```python
from build123d import *
from OCP.BRepFilletAPI import BRepFilletAPI_MakeChamfer

# Parameters (mm, degrees)
SCHIZZO1_W                   = 34
SCHIZZO1_H                   = 30
ESTRUSIONE_ESTRUSIONE1_DEPTH = 22
SCHIZZO2_W                   = 1
SCHIZZO2_H                   = 14.267949192
TAGLIO_ESTRUSIONE1_DEPTH     = 37.193922142
SCHIZZO3_W                   = 10.8571
SCHIZZO3_H                   = 4
TAGLIO_ESTRUSIONE2_DEPTH     = 37.193922142
SCHIZZO4_W                   = 11.8571
SCHIZZO4_H                   = 4
TAGLIO_ESTRUSIONE3_DEPTH     = 37.193922142
SCHIZZO5_W                   = 1
SCHIZZO5_H                   = 10.267949192
TAGLIO_ESTRUSIONE4_DEPTH     = 37.193922142
SCHIZZO6_W                   = 15.2
SCHIZZO6_H                   = 0.4
TAGLIO_ESTRUSIONE5_DEPTH     = 37.193922142
SFORMO1_ANGLE                = 60
SFORMO2_ANGLE                = 60
SFORMO3_ANGLE                = 45
SFORMO4_ANGLE                = 45
SMUSSO1_SIZE                 = 0.230940108
SMUSSO1_SIZE2                = 0.4
SMUSSO2_SIZE                 = 0.379
SMUSSO3_SIZE                 = 1


with BuildPart() as part:
    # Schizzo1 → Estrusione-Estrusione1 (new body)
    with BuildSketch(Plane(origin=(0, 11, 0), x_dir=(1, 0, 0), z_dir=(0, 1, 0))):
        with Locations((0, -15)):
            Rectangle(SCHIZZO1_W, SCHIZZO1_H)
    extrude(amount=-ESTRUSIONE_ESTRUSIONE1_DEPTH)

    # Schizzo2 → Taglio-Estrusione1 (cut, through all)
    with BuildSketch(Plane.XY.offset(30)):
        with Locations((16.5, -3.866025404)):
            Rectangle(SCHIZZO2_W, SCHIZZO2_H)
    extrude(amount=-TAGLIO_ESTRUSIONE1_DEPTH, mode=Mode.SUBTRACT)

    # Schizzo3 → Taglio-Estrusione2 (cut, through all)
    with BuildSketch(Plane.XY.offset(30)):
        with Locations((10.57145, -9)):
            Rectangle(SCHIZZO3_W, SCHIZZO3_H)
    extrude(amount=-TAGLIO_ESTRUSIONE2_DEPTH, mode=Mode.SUBTRACT)

    # Schizzo4 → Taglio-Estrusione3 (cut, through all)
    with BuildSketch(Plane.XY.offset(30)):
        with Locations((-11.07145, -9)):
            Rectangle(SCHIZZO4_W, SCHIZZO4_H)
    extrude(amount=-TAGLIO_ESTRUSIONE3_DEPTH, mode=Mode.SUBTRACT)

    # Schizzo5 → Taglio-Estrusione4 (cut, through all)
    with BuildSketch(Plane.XY.offset(30)):
        with Locations((-16.5, -1.866025404)):
            Rectangle(SCHIZZO5_W, SCHIZZO5_H)
    extrude(amount=-TAGLIO_ESTRUSIONE4_DEPTH, mode=Mode.SUBTRACT)

    # Schizzo6 → Taglio-Estrusione5 (cut, through all)
    with BuildSketch(Plane.XY.offset(30)):
        with Locations((0, 10.8)):
            Rectangle(SCHIZZO6_W, SCHIZZO6_H)
    extrude(amount=-TAGLIO_ESTRUSIONE5_DEPTH, mode=Mode.SUBTRACT)

    # Sformo1
    sformo1_faces = [part.faces().sort_by_distance(p)[0] for p in [
        (16.5, 3.267949192, 15),
    ]]
    draft(sformo1_faces, Plane(origin=(16, 3.267949192, 0), x_dir=(0, 0, 1), z_dir=(1, 0, 0)), SFORMO1_ANGLE)

    # Sformo2
    sformo2_faces = [part.faces().sort_by_distance(p)[0] for p in [
        (-16.5, 3.267949192, 15),
    ]]
    draft(sformo2_faces, Plane(origin=(-16, -7, 0), x_dir=(0, 0, -1), z_dir=(-1, 0, 0)), SFORMO2_ANGLE)

    # Sformo3
    sformo3_faces = [part.faces().sort_by_distance(p)[0] for p in [
        (5.1429, -9, 15),
        (-5.1429, -9, 15),
    ]]
    draft(sformo3_faces, Plane(origin=(0, -11, 0), x_dir=(0, 0, -1), z_dir=(0, -1, 0)), SFORMO3_ANGLE)

    # Sformo4
    sformo4_faces = [part.faces().sort_by_distance(p)[0] for p in [
        (-7.6, 10.8, 15),
        (7.6, 10.8, 15),
    ]]
    draft(sformo4_faces, Plane(origin=(-7.6, 10.6, 0), x_dir=(1, 0, 0), z_dir=(0, 1, 0)), SFORMO4_ANGLE)

    # Schizzo7 → Taglia-Rivoluzione1 (revolve, cut)
    with BuildSketch(Plane.XZ, mode=Mode.PRIVATE) as taglia_rivoluzione1_sk:
        Polygon((7.5, 30), (0, 30), (0, 0), (7.5, 0), (7.5, 2), (7.85, 2), (7.85, 3.15), (7.5, 3.15), (7.5, 26.85), (7.85, 26.85), (7.85, 28), (7.5, 28), align=None)
    revolve(taglia_rivoluzione1_sk.sketch.rotate(Axis((0, 0, 30), (0, 0, -1)), 180), axis=Axis((0, 0, 30), (0, 0, -1)), mode=Mode.SUBTRACT)

    # Schizzo8 → Taglia-Rivoluzione2 (revolve, cut)
    with BuildSketch(Plane.XY.offset(6), mode=Mode.PRIVATE) as taglia_rivoluzione2_sk:
        Polygon((-10.379, 11), (-12, 11), (-12, -7), (-10.3, -7), (-10.3, 3), (-10.379, 3), align=None)
    revolve(taglia_rivoluzione2_sk.sketch.rotate(Axis((-12, 11, 6), (0, -1, 0)), 270), axis=Axis((-12, 11, 6), (0, -1, 0)), mode=Mode.SUBTRACT)

    # Schizzo9 → Taglia-Rivoluzione3 (revolve, cut)
    with BuildSketch(Plane.XY.offset(24), mode=Mode.PRIVATE) as taglia_rivoluzione3_sk:
        Polygon((-10.379, 11), (-12, 11), (-12, -7), (-10.3, -7), (-10.3, 3), (-10.379, 3), align=None)
    revolve(taglia_rivoluzione3_sk.sketch.rotate(Axis((-12, 11, 24), (0, -1, 0)), 270), axis=Axis((-12, 11, 24), (0, -1, 0)), mode=Mode.SUBTRACT)

    # Schizzo10 → Taglia-Rivoluzione4 (revolve, cut)
    with BuildSketch(Plane.XY.offset(6), mode=Mode.PRIVATE) as taglia_rivoluzione4_sk:
        Polygon((13.621, 11), (12, 11), (12, -7), (13.7, -7), (13.7, 3), (13.621, 3), align=None)
    revolve(taglia_rivoluzione4_sk.sketch.rotate(Axis((12, 11, 6), (0, -1, 0)), 270), axis=Axis((12, 11, 6), (0, -1, 0)), mode=Mode.SUBTRACT)

    # Schizzo11 → Taglia-Rivoluzione5 (revolve, cut)
    with BuildSketch(Plane.XY.offset(24), mode=Mode.PRIVATE) as taglia_rivoluzione5_sk:
        Polygon((13.621, 11), (12, 11), (12, -7), (13.7, -7), (13.7, 3), (13.621, 3), align=None)
    revolve(taglia_rivoluzione5_sk.sketch.rotate(Axis((12, 11, 24), (0, -1, 0)), 270), axis=Axis((12, 11, 24), (0, -1, 0)), mode=Mode.SUBTRACT)

    # Smusso1: one chamfer whose edges measure the first distance from different faces: ONE call of the kernel's chamfer builder (chamfer() names one face for all edges)
    smusso1_edges_1 = [part.edges().sort_by_distance(p)[0] for p in [
        (-12, -7, 7.7),
        (-12, -7, 25.7),
    ]]
    smusso1_side_1 = [part.faces().sort_by_distance(p)[0] for p in [
        (-12.626775869, -7, 15),
    ]]
    smusso1_edges_2 = [part.edges().sort_by_distance(p)[0] for p in [
        (12, -7, 7.7),
        (12, -7, 25.7),
    ]]
    smusso1_side_2 = [part.faces().sort_by_distance(p)[0] for p in [
        (12.626775869, -7, 15),
    ]]
    smusso1 = BRepFilletAPI_MakeChamfer(part.part.solid().wrapped)
    for e in smusso1_edges_1:
        smusso1.Add(SMUSSO1_SIZE, SMUSSO1_SIZE2, e.wrapped, smusso1_side_1[0].wrapped)  # the first distance lies on this face
    for e in smusso1_edges_2:
        smusso1.Add(SMUSSO1_SIZE, SMUSSO1_SIZE2, e.wrapped, smusso1_side_2[0].wrapped)  # the first distance lies on this face
    add(Compound.cast(smusso1.Shape()), mode=Mode.REPLACE)

    # Smusso2
    smusso2_edges = [part.edges().sort_by_distance(p)[0] for p in [
        (-12, 11, 7.621),
        (-12, 11, 25.621),
        (12, 11, 7.621),
        (12, 11, 25.621),
        (-12.5, 11, 30),
        (12.5, 11, 0),
        (-12.5, 11, 0),
        (12.5, 11, 30),
    ]]
    chamfer(smusso2_edges, length=SMUSSO2_SIZE)

    # Smusso3
    smusso3_edges = [part.edges().sort_by_distance(p)[0] for p in [
        (17, 11, 15),
        (-17, 11, 15),
    ]]
    chamfer(smusso3_edges, length=SMUSSO3_SIZE)


solid = part.part
```
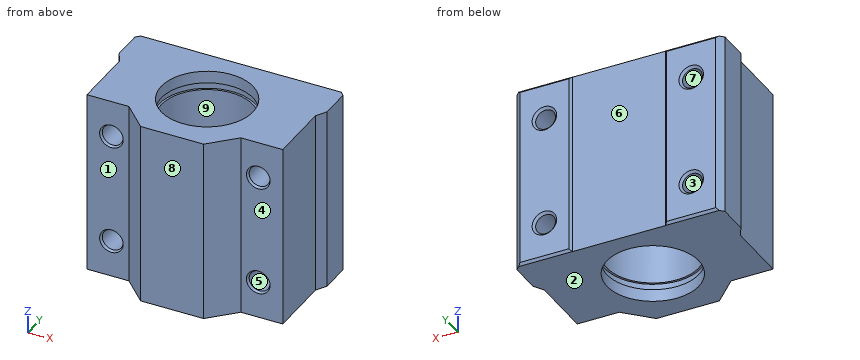
Geometry check sheet. Reference: the model listing, model coordinates, mm. Face numbers are marked on the shaded views. A direction names the side the tool comes from. Coordinates: 2 decimals unless noted, no trailing zeros. Write each loop counter-clockwise with the first axis right and the second up, starting at its lowest first coordinate (ties: lowest second). Pieces come first, ordered by that corner, then holes. Notation, with made-up numbers: M -10,6 L 24,6 A3 ccw 24,11 Z; hole C 26,7 d10. An arc over 180 degrees is marked long. Answer as a JSON object with one key per item and string values.
1. Scan lines: L1, parallel to Z at x = -7.5, y = -1.25; L2, parallel to Z at x = -11.5, y = 5.25; L3, parallel to X at y = 1.75, z = 23.5. Record each from-to range of solid material in increasing order.
Answers below:
{"L1": "z = 0 to 2, 3.15 to 26.85, 28 to 30", "L2": "z = 0 to 4.46, 7.54 to 22.46, 25.54 to 30", "L3": "x = -16 to -13.62, -10.38 to -7.29, 7.29 to 10.38, 13.62 to 16"}
2. Section check A-A, the plane x = 0. Enter the section's corners in (y, z).
Answers below:
{"outline": "M -11,0 L -7.5,0 L -7.5,2 L -7.85,2 L -7.85,3.15 L -7.5,3.15 L -7.5,26.85 L -7.85,26.85 L -7.85,28 L -7.5,28 L -7.5,30 L -11,30 Z; M 7.5,0 L 10.6,0 L 10.6,30 L 7.5,30 L 7.5,28 L 7.85,28 L 7.85,26.85 L 7.5,26.85 L 7.5,3.15 L 7.85,3.15 L 7.85,2 L 7.5,2 Z"}
3. Draft check along Y on the marked faces 6, 7, 8 and 9. Enter one of: released by +Y, released by -Y, zero draft, split by the parting line, or undercut.
Answers below:
{"face 6": "released by +Y", "face 7": "zero draft", "face 8": "released by -Y", "face 9": "undercut"}
4. Section check D-D, the plane z = 17.5. Enter the section's corners in (x, y).
Answers below:
{"outline": "M -17,5 L -16,3.27 L -16,-7 L -9.14,-7 L -5.14,-11 L 5.14,-11 L 9.14,-7 L 16,-7 L 16,3.27 L 17,5 L 17,10 L 16,11 L 8,11 L 7.6,10.6 L -7.6,10.6 L -8,11 L -16,11 L -17,10 Z; hole C 0,0 d15"}
5. Go/stop test with flat-tipped pins: pin 1 Ø3 at (y, z) = (-2.5, 7.5) entering from -X; pin 2 Ø3.5 at (x, z) = (13, 20) entering from -Y; pin 3 Ø4 at (y, z) = (-2, 17) entering from +X. Record where each tip stops, or that it passes through.
Answers below:
{"pin 1": "stops at x = -16", "pin 2": "stops at y = -7", "pin 3": "stops at x = 16"}
6. Section check B-B, the plane y = 2.25. Enter the section's corners in (x, z), plus the area to 3 significant figures.
Answers below:
{"outline": "M -16,0 L -7.15,0 L -7.15,2 L -7.52,2 L -7.52,3.15 L -7.15,3.15 L -7.15,26.85 L -7.52,26.85 L -7.52,28 L -7.15,28 L -7.15,30 L -16,30 Z; M 7.15,0 L 16,0 L 16,30 L 7.15,30 L 7.15,28 L 7.52,28 L 7.52,26.85 L 7.15,26.85 L 7.15,3.15 L 7.52,3.15 L 7.52,2 L 7.15,2 Z; hole C -12,6 d3.4; hole C -12,24 d3.4; hole C 12,6 d3.4; hole C 12,24 d3.4", "area": "493 mm²"}
7. Section check C-C, the plane x = 12. Give the number of separate pieces and of enclosed holes in the cut face, plus the area to 3 significant figures.
Answers below:
{"separate pieces": "3", "enclosed holes": "0", "area": "420 mm²"}
8. Tool access check on the marked faces 1, 2, 3, 4 and 5. Record the directions out of +Z, -Z, +X, -X, +Y, -Y that give a thin tool (end or side, any length) a straight path to the whole face; none if there is none.
Answers below:
{"face 1": "+Z, -Z, -X, -Y", "face 2": "-Z, +X, -X, +Y, -Y", "face 3": "+Y, -Y", "face 4": "+Z, -Z, +X, -Y", "face 5": "-Y"}
